Autodesk Inventor part; units mm, degrees
ref_plane "YZ Plane" through (0, 0, 0) normal (1, 0, 0) x (0, 1, 0)
ref_plane "XZ Plane" through (0, 0, 0) normal (0, 1, 0) x (-1, 0, 0)
ref_plane "XY Plane" through (0, 0, 0) normal (0, 0, 1) x (1, 0, 0)
sketch "Esboço1" plane through (0, 0, 0) normal (0, 0, 1) x (1, 0, 0)
  line L0 (-293, 0) -> (-323, 0) construction
  line L1 (-323, 0) -> (-323, 50) construction
  line L2 (27, 0) -> (27, 50) construction
  line L3 (27, 0) -> (0, 0) construction
  line L4 (-3, 50) -> (27, 50) construction
  line L5 (-323, 50) -> (-293, 50) construction
  line L6 (27, 0) -> (-323, 0)
  line L7 (-323, 0) -> (-323, 50)
  line L8 (-323, 50) -> (27, 50)
  line L9 (27, 50) -> (27, 0)
extrude "bloco principal" add sketch "Esboço1" along normal blind 10.5
sketch "Esboço4" plane through (0, 0, 10.5) normal (0, 0, 1) x (1, 0, 0)
  line L0 (27, 0) -> (27, 50)
  line L1 (27, 40) -> (-323, 40) construction
  line L2 (-323, 50) -> (-323, 0)
  line L3 (5.5, 40) -> (-145.5, 40) construction
  line L4 (1.5, 44) -> (-141.5, 44)
  line L5 (-141.5, 36) -> (1.5, 36)
  arc A0 (1.5, 36) -> (1.5, 44) centre (1.5, 40) ccw
  arc A1 (-141.5, 44) -> (-141.5, 36) centre (-141.5, 40) ccw
  line L6 (-150.5, 40) -> (-301.5, 40) construction
  line L7 (-154.5, 44) -> (-297.5, 44)
  line L8 (-297.5, 36) -> (-154.5, 36)
  arc A2 (-154.5, 36) -> (-154.5, 44) centre (-154.5, 40) ccw
  arc A3 (-297.5, 44) -> (-297.5, 36) centre (-297.5, 40) ccw
  line L9 (-323, 0) -> (27, 0)
  line L10 (27, 50) -> (-323, 50)
  point P0 (0, 0)
  point P1 (-70, 40)
  point P2 (-226, 40)
  dimension "d39" = 97
  dimension "d40" = 97
  dimension "d41" = 8
  dimension "d42" = 8
  dimension "d43" = 143
  dimension "d44" = 143
  dimension "d46" = 10
extrude "fenda" cut sketch "Esboço4" against normal through all contours A0 L5 A1 L4 | A2 L8 A3 L7
sketch "Esboço5" plane through (0, 0, 10.5) normal (0, 0, 1) x (1, 0, 0)
  line L0 (27, 0) -> (27, 50)
  line L1 (27, 17) -> (-323, 17) construction
  line L2 (-323, 50) -> (-323, 0)
  circle A0 centre (-148, 17) radius 12.5
  circle A1 centre (-213, 17) radius 12.5
  circle A2 centre (-278, 17) radius 12.5
  circle A3 centre (-83, 17) radius 12.5
  circle A4 centre (-148, 17) radius 12.5 construction
  circle A5 centre (-213, 17) radius 12.5 construction
  circle A6 centre (-18, 17) radius 12.5
  circle A7 centre (-83, 17) radius 12.5 construction
  circle A8 centre (-148, 17) radius 12.5 construction
  line L3 (-323, 0) -> (27, 0)
  point P0 (0, 0)
  dimension "d51" = 65
  dimension "d54" = 65
  dimension "d57" = 17
  dimension "d58" = 25
extrude "furos traseiros" cut sketch "Esboço5" against normal through all
sketch "Esboço6" plane through (0, 0, 10.5) normal (0, 0, 1) x (1, 0, 0)
  circle A0 centre (-308, 12.5) radius 1.621 construction
  circle A1 centre (-308, 37.5) radius 1.621 construction
  circle A2 centre (12, 12.5) radius 1.621 construction
  circle A3 centre (12, 37.5) radius 1.621 construction
  point P0 (0, 0)
hole "furos fixação" at (-308, 12.5, 10.5) at (-308, 37.5, 10.5) at (12, 12.5, 10.5) at (12, 37.5, 10.5) direction (0, 0, -1) diameter 4 end through all counterbore diameter 8 counterbore depth 4.5
chamfer "Chanfro1" distance 1 angle 45 4 edges at (27, 0, 5.25) (27, 50, 5.25) (-323, 50, 5.25) (-323, 0, 5.25)
equation "\"d41\" = d42"
equation "\"d44\" = d43"
properties part number "SuportePincasBlocoFabricado"
Here's how the part is built. I have some questions about the finished solid (model axes, mm). A direction names the side the tool comes from. Coordinates: 2 decimals unless noted, no trailing zeros. Order: outer loops, then holes, each group sorted by start corner. A loop starts at its lowest first (then second) coordinate and runs counter-clockwise, first axis right, second up. Notation, with made-up numbers: (89.25, 15) - (134.25, 15) arc R17 ccw to (134.25, 33) - close; hole circle Ø7 at (7.25, -9.5). An arc over 180 degrees is marked (long way). One line per question, with ' | ' between items. Start each with the question number.
1. If we mould it in two halves opening along X, with no side actions, what happens to faces 1 (the flat face through (-150, 50, 5)), 2 (the flat face through (-227, 36, 5))? For each: released by +X, released by -X, zero draft, split by the parting line, or undercut.
2. If we section it at D-D (x = -286): Write out the boundary of the cut face in (y, z).
3. If we section it at C-C (z = 2.25): Give the number of separate pieces and of enclosed holes in the cut face, and give its area (3 significant figures).
4. Please list where these lines run through material, in increasing order: line 1 along Y through (x, z) = (-308, 2.6); line 2 along Y through (x, z) = (12, 8.85); line 3 along Y through (x, z) = (-115, 9). Write a range as [from, to].
5. Which directions (+Z, -Z, +X, -X, +Y, -Y) give clear straight access to the entire face, cutting with the end or side of a thin tool? Please do faces 3 (the cylindrical face through (-301.5, 40.1, 5.3)), 4 (the flat face through (-306, 11, 6)), 5 (the flat face through (-150, 31, 0)).
6. I'm going to push flat-ended pins straight in: pin 1 Ø10.5 at (x, y) = (-308, 37.5) entering from -Z; pin 2 Ø4 at (x, y) = (10.5, 12.5) entering from +Z. Where does each tip first touch, or does it pass through?
7. If we section it at B-B (x = -213): Write out the boundary of the cut face in (y, z), and give its area (4 significant figures).
8. If we section it at A-A (x = -44.5): Write out the boundary of the cut face in (y, z), and give its area (3 significant figures).
Model answer:
1) face 1: zero draft | face 2: undercut
2) outline: (0, 0) - (7.4, 0) - (7.4, 10.5) - (0, 10.5) - close; (26.6, 0) - (36, 0) - (36, 10.5) - (26.6, 10.5) - close; (44, 0) - (50, 0) - (50, 10.5) - (44, 10.5) - close
3) separate pieces: 1 | enclosed holes: 11 | area: 12,600 mm²
4) line 1: y = [0, 10.5], [14.5, 35.5], [39.5, 50] | line 2: y = [0, 8.5], [16.5, 33.5], [41.5, 50] | line 3: y = [0, 36], [44, 50]
5) face 3: +Z, -Z | face 4: +Z | face 5: -Z, +X, -X, +Y, -Y
6) pin 1: stops at z = 0 | pin 2: stops at z = 6
7) outline: (0, 0) - (4.5, 0) - (4.5, 10.5) - (0, 10.5) - close; (29.5, 0) - (36, 0) - (36, 10.5) - (29.5, 10.5) - close; (44, 0) - (50, 0) - (50, 10.5) - (44, 10.5) - close | area: 178.5 mm²
8) outline: (0, 0) - (36, 0) - (36, 10.5) - (0, 10.5) - close; (44, 0) - (50, 0) - (50, 10.5) - (44, 10.5) - close | area: 441 mm²
